Geometry check sheet. Reference: the model listing, model coordinates, mm. A direction names the side the tool comes from. Round coordinates to 2 decimals unless told otherwise and drop trailing zeros. Loops run counter-clockwise (first coordinate to the right, second up) from the corner with the lowest first, then second, coordinate; pieces in that order, holes last. Notation, with made-up numbers: (50, 42) -> (78, 42) arc R14 ccw to (78, 65) -> close; hole circle Ø8 at (-37.5, 20.5). An arc over 180 degrees is marked (long way). Use a Markdown table: item, result. Add a question column.
Q1. Material ranges on L1, parallel to Y at x = 153, z = 5; L2, parallel to Y at x = 138.5, z = 5.75; L3, parallel to Y at x = 154.5, z = 2.75, recorded low to high.
Q2. Sectioned sample at A-A, the plane y = 13. Enter the section's corners in (x, z), then the cut area to 3 significant figures.
Q3. Sectioned sample at B-B, the plane z = 2.25. Give the number of separate pieces and of enclosed holes in the cut face, then the cut area to 3 significant figures.
Q4. Set-up check for faces 1 (the face through (201.317, -45.675, 3.131)), 2 (the face through (208.753, 169.347, 3.219)): record each of +Z, -Z, +X, -X, +Y, -Y from which the full face is reachable in a straight line by a thin tool's end or side.
Q5. Release check for a two-part mould opening along X. For faces 3 (the face through (200, 80, 6.35)), 4 (the face through (249.952, -48, 3)), 5 (the face through (184.7, -42.87, 3.13)) record: released by +X, released by -X, zero draft, split by the parting line, or undercut.
Q6. Gauge pin test, flat ends, axial feed: P1, Ø0.7, axis at x = 248, z = 3.5, coming from the +Y side; P2, Ø1, axis at x = 220, y = 67.5, coming from the -Z side; P3, Ø3, axis at x = 165, z = 2.5, coming from the +Y side; P4, Ø2, axis at y = 151.5, z = 3.5, coming from the -X side. Record the tip position at first contact, or that the pin passes through.
```python
from build123d import *

# Parameters (mm, degrees)
SKETCH1_R           = 2.6289
SKETCH1_R_2         = 2.667
SKETCH1_R_3         = 3.2639
BOSS_EXTRUDE1_DEPTH = 6.35
SKETCH3_R           = 14.5542
SKETCH3_R_2         = 3.2639
SKETCH3_R_3         = 2.6289
BOSS_EXTRUDE2_DEPTH = 6.35
SKETCH4_R           = 14.5542
SKETCH4_R_2         = 2.0193
CUT_EXTRUDE1_DEPTH  = 7.35
BOSS_EXTRUDE3_DEPTH = 6.35
FILLET1_R           = 4.7625
FILLET2_R           = 4.7625


with BuildPart() as part:
    # Sketch1 → Boss-Extrude1 (new body)
    with BuildSketch(Plane.XY):
        with BuildLine():
            Line((176.178529946, -50.8), (240.761529124, -50.8))
            ThreePointArc((240.761529124, -50.8), (235.877364624, 70.061564101), (173.992462346, 173.992462346))
            Line((173.992462346, 173.992462346), (129.652447748, 129.652447748))
            ThreePointArc((129.652447748, 129.652447748), (169.399086533, 70.167399096), (183.35625, 0))
            ThreePointArc((183.35625, 0), (181.552952325, -25.652288715), (176.178529946, -50.8))
        make_face()
        with Locations((191.177219016, 6.676055597)):
            Circle(SKETCH1_R, mode=Mode.SUBTRACT)
        with Locations((156.698666372, 109.721587421)):
            Circle(SKETCH1_R, mode=Mode.SUBTRACT)
        with Locations((176.732380322, 73.20494884)):
            Circle(SKETCH1_R_2, mode=Mode.SUBTRACT)
        with Locations((186.787775735, -41.275)):
            Circle(SKETCH1_R, mode=Mode.SUBTRACT)
        with Locations((238.125, 0)):
            Circle(SKETCH1_R_3, mode=Mode.SUBTRACT)
        with Locations((234.507346186, 41.349972307)):
            Circle(SKETCH1_R_3, mode=Mode.SUBTRACT)
        with Locations((223.764305325, 81.443546629)):
            Circle(SKETCH1_R_3, mode=Mode.SUBTRACT)
        with Locations((206.222299276, 119.0625)):
            Circle(SKETCH1_R_3, mode=Mode.SUBTRACT)
        with Locations((182.414333018, 153.063799557)):
            Circle(SKETCH1_R_3, mode=Mode.SUBTRACT)
        with Locations((234.507346186, -41.349972307)):
            Circle(SKETCH1_R_3, mode=Mode.SUBTRACT)
        with BuildLine():
            ThreePointArc((202.946, 0), (201.859935486, -20.967721902), (198.61336608, -41.711026485))
            ThreePointArc((198.61336608, -41.711026485), (201.391341659, -45.688667392), (205.368929989, -42.910616532))
            ThreePointArc((205.368929989, -42.910616532), (208.692287116, -21.569601625), (209.804, 0))
            ThreePointArc((209.804, 0), (198.481076932, 67.99250338), (165.734482585, 128.646024805))
            ThreePointArc((165.734482585, 128.646024805), (160.923178893, 129.252192093), (160.317011605, 124.440888401))
            ThreePointArc((160.317011605, 124.440888401), (191.993196693, 65.769988136), (202.946, 0))
        make_face(mode=Mode.SUBTRACT)
    extrude(amount=BOSS_EXTRUDE1_DEPTH)

    # Sketch3 → Boss-Extrude2 (add)
    with BuildSketch(Plane.XY.offset(6.35)):
        with BuildLine():
            Line((129.652447748, 129.652447748), (161.644610179, 161.644610179))
            Line((161.644610179, 161.644610179), (173.992462346, 173.992462346))
            ThreePointArc((173.992462346, 173.992462346), (187.203995727, 159.691633751), (199.243521921, 144.391041546))
            Line((199.243521921, 144.391041546), (208.072252438, 163.324315239))
            ThreePointArc((208.072252438, 163.324315239), (208.734128286, 169.432705073), (205.528624059, 174.674388835))
            Line((205.528624059, 174.674388835), (168.450190134, 205.497612521))
            ThreePointArc((168.450190134, 205.497612521), (163.856747392, 207.579840958), (158.844030643, 207.024807371))
            Line((158.844030643, 207.024807371), (137.554097629, 198.565416651))
            ThreePointArc((137.554097629, 198.565416651), (127.316076149, 190.310286973), (123.536791738, 177.713411997))
            Line((123.536791738, 177.713411997), (123.841133335, 143.507548105))
            ThreePointArc((123.841133335, 143.507548105), (125.38482655, 136.008742521), (129.652447748, 129.652447748))
        make_face()
        with Locations((145.760912093, 177.911147809)):
            Circle(SKETCH3_R, mode=Mode.SUBTRACT)
        with Locations((199.439670766, 167.349754182)):
            Circle(SKETCH3_R_2, mode=Mode.SUBTRACT)
        with Locations((162.361236841, 198.172977868)):
            Circle(SKETCH3_R_2, mode=Mode.SUBTRACT)
        with Locations((128.876648593, 161.759110908)):
            Circle(SKETCH3_R_3, mode=Mode.SUBTRACT)
    extrude(amount=-BOSS_EXTRUDE2_DEPTH)

    # Sketch4 → Cut-Extrude1 (cut, through all)
    with BuildSketch(Plane.XY.offset(6.35)):
        with Locations((143.684097937, 143.684097937)):
            Circle(SKETCH4_R)
        with Locations((157.154482119, 157.154482119)):
            Circle(SKETCH4_R_2)
        with Locations((148.614600746, 125.283210946)):
            Circle(SKETCH4_R_2)
    extrude(amount=-CUT_EXTRUDE1_DEPTH, mode=Mode.SUBTRACT)

    # Sketch5 → Boss-Extrude3 (add)
    with BuildSketch(Plane.XY.offset(6.35)):
        with BuildLine():
            Line((240.761529124, -50.8), (249.951861983, -50.8))
            Line((249.951861983, -50.8), (249.951861983, -44.45))
            Line((249.951861983, -44.45), (242.014361983, -44.45))
            ThreePointArc((242.014361983, -44.45), (241.408825198, -47.629119481), (240.761529124, -50.8))
        make_face()
    extrude(amount=-BOSS_EXTRUDE3_DEPTH)

    # Fillet1
    fillet1_edges = [part.edges().sort_by_distance(p)[0] for p in [
        (242.014361983, -44.45, 3.175),
    ]]
    fillet(fillet1_edges, radius=FILLET1_R)

    # Fillet2
    fillet2_edges = [part.edges().sort_by_distance(p)[0] for p in [
        (199.243521921, 144.391041546, 3.175),
    ]]
    fillet(fillet2_edges, radius=FILLET2_R)


solid = part.part
```
Values:
| question | item | result |
|---|---|---|
| 1 | L1 | 101.05 to 132.5, 154.87 to 165.28, 190.54 to 204.7 |
| 1 | L2 | 120.16 to 130.08, 157.28 to 165.3, 190.52 to 198.94 |
| 1 | L3 | 98.74 to 108.28, 111.16 to 133.95, 153.42 to 166.27, 189.55 to 205.3 |
| 2 | outline | (182.89, 0) -> (202.53, 0) -> (202.53, 6.35) -> (182.89, 6.35) -> close; (209.4, 0) -> (245.72, 0) -> (245.72, 6.35) -> (209.4, 6.35) -> close |
| 2 | area | 355 mm^2 |
| 3 | separate pieces | 1 |
| 3 | enclosed holes | 18 |
| 3 | area | 14,400 mm^2 |
| 4 | face 1 | +Z, -Z |
| 4 | face 2 | +Z, -Z, +X |
| 5 | face 3 | zero draft |
| 5 | face 4 | released by +X |
| 5 | face 5 | undercut |
| 6 | P1 | y = -44.45 |
| 6 | P2 | z = 0 |
| 6 | P3 | y = 207.63 |
| 6 | P4 | x = 123.76 |
